Geometry: final body of the model. Coordinates: model frame, mm. A direction names the side the tool comes from. Give positions to 0.01 mm unless a question says otherwise; leave off trailing zeros. Loops run counter-clockwise (first coordinate to the right, second up) from the corner with the lowest first, then second, coordinate; pieces in that order, holes last. Notation, with made-up numbers: (34, 70.5) -> (77, 70.5) arc R23 cw to (77, 105.5) -> close; hole circle Ø7 at (-33.5, 14.25). An arc over 180 degrees is marked (long way). Answer in a Markdown table with one row per item. Add a question column.
1) Section query D-D (y = 31). Return the cut outline in (x, z), plus the area to 3 significant figures.
2) Draft query along Z for faces 1 (the flat face through (15, -15, 177.3)), 2 (the flat face through (15, -15, 190)), 3 (the flat face through (-15, -15, -190)), 4 (the cylindrical face through (-27.715, -21.251, 183.739)). Return one class per face: +Z half, -Z half, draft (parallel to the pull), parting line (faces both ways), or undercut.
3) Section query C-C (z = -25.5). Return the cut outline in (x, y).
4) Section query A-A (x = 0). Return the cut outline in (y, z) (3 decimals).
5) Line query: line 1 (Y direction, x = 0, z = 72); line 2 (Z direction, x = -14, y = -15.5); line 3 (X direction, y = -2.5, z = -78). Output: solid intervals per line, ascending. Write a range as from..to.
6) Access query for faces 5 (the cylindrical face through (-27.715, 21.251, -183.739)), 6 (the cylindrical face through (-15.12, 11.59, -2.48)). Directions: +Z, -Z, +X, -X, +Y, -Y. A direction counts if a zero-diameter tool reaches every point of the face in a straight line with its end or side. Return the directions, or none.
7) First-contact query: P1, Ø1.5, axis at y = -11.5, z = 132, coming from the -X side; P2, Ø5, axis at x = 15.5, z = -9, coming from the -Y side; P3, Ø12, axis at x = -4, z = -95, coming from the +Y side. Flat tips, straight axial feed; report the tip coordinate or a pass-through.
Autodesk Inventor part; units mm, degrees
ref_plane "YZ Plane" through (0, 0, 0) normal (1, 0, 0) x (0, 1, 0)
ref_plane "XZ Plane" through (0, 0, 0) normal (0, 1, 0) x (-1, 0, 0)
ref_plane "XY Plane" through (0, 0, 0) normal (0, 0, 1) x (1, 0, 0)
sketch "Sketch1" plane through (0, 0, 0) normal (0, 0, 1) x (1, 0, 0)
  circle A0 centre (0, 0) radius 19.05
  circle A1 centre (0, 0) radius 18.288
  dimension "d6" = 38.1
  dimension "d9" = 36.576
extrude "Extrusion1" add sketch "Sketch1" along normal mid plane 380
sketch "Sketch2" plane through (0, 0, 190) normal (0, 0, 1) x (1, 0, 0)
  circle A0 centre (0, 0) radius 34.925
  circle A1 centre (0, 0) radius 19.05
  dimension "d10" = 69.85
extrude "Extrusion2" add sketch "Sketch2" against normal blind 12.7
mirror "Mirror1" about plane through (0, 0, 0) normal (0, 0, 1) of "Extrusion2"
equation "\"d7\" = Length"
equation "\"Length\" = 380"
properties part number "Pipe300"
Evaluation:
| question | item | result |
|---|---|---|
| 1 | outline | (-16.09, -190) -> (16.09, -190) -> (16.09, -177.3) -> (-16.09, -177.3) -> close; (-16.09, 177.3) -> (16.09, 177.3) -> (16.09, 190) -> (-16.09, 190) -> close |
| 1 | area | 817 mm² |
| 2 | face 1 | undercut |
| 2 | face 2 | +Z half |
| 2 | face 3 | -Z half |
| 2 | face 4 | draft |
| 3 | outline | circle Ø38.1 at (0, 0); hole circle Ø36.58 at (0, 0) |
| 4 | outline | (-34.925, -190) -> (-18.288, -190) -> (-18.288, 190) -> (-34.925, 190) -> (-34.925, 177.3) -> (-19.05, 177.3) -> (-19.05, -177.3) -> (-34.925, -177.3) -> close; (18.288, -190) -> (34.925, -190) -> (34.925, -177.3) -> (19.05, -177.3) -> (19.05, 177.3) -> (34.925, 177.3) -> (34.925, 190) -> (18.288, 190) -> close |
| 5 | line 1 | -19.05..-18.29, 18.29..19.05 |
| 5 | line 2 | -190..-177.3, 177.3..190 |
| 5 | line 3 | -18.89..-18.12, 18.12..18.89 |
| 6 | face 5 | +Z, -Z |
| 6 | face 6 | none |
| 7 | P1 | x = -15.73 |
| 7 | P2 | y = -13.92 |
| 7 | P3 | y = 19.05 |
